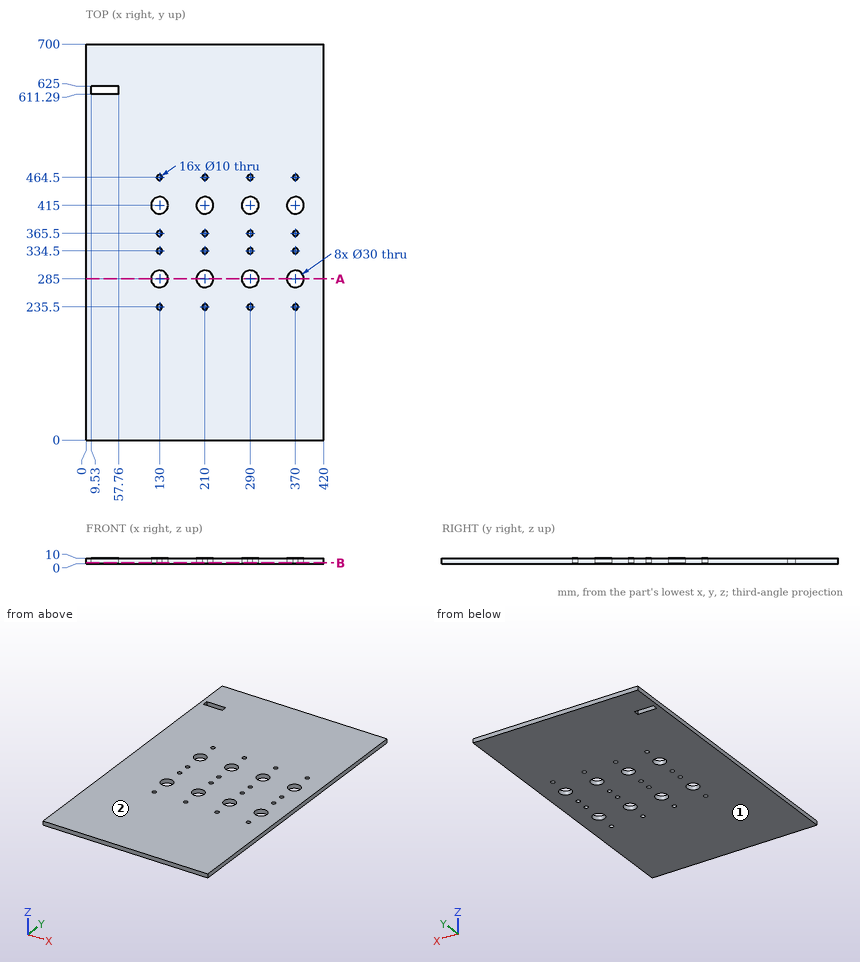
Answer from the drawing. Dimensions are ordinates in mm from the lowest x, y and z of the part. Give positions to 0.01 mm unless a question says otherwise; leave off trailing zeros. Order: outer loops, then holes, each group sorted by start corner. A loop starts at its lowest first (then second) coordinate and runs counter-clockwise, first axis right, second up.
Item 1: The part is cut by section A-A, the plane y = 285. Give the vertices of the cut face in (x, z), and give its area (3 significant figures).
From the geometry:
outline: (0, 0) - (115, 0) - (115, 10) - (0, 10) - close; (145, 0) - (195, 0) - (195, 10) - (145, 10) - close; (225, 0) - (275, 0) - (275, 10) - (225, 10) - close; (305, 0) - (355, 0) - (355, 10) - (305, 10) - close; (385, 0) - (420, 0) - (420, 10) - (385, 10) - close
area: 3,000 mm2
Item 2: For a pull along Z with two mould halves and no side action, classify the marked faces 1 and 2 as pulls with the +Z half, pulls with the -Z half, needs draft (parallel to the pull), parting line crosses it, or undercut.
From the geometry:
face 1: pulls with the -Z half
face 2: pulls with the +Z half
Item 3: Find the intervals of material crossed by probe 1 along X at (y, z) = (334.5, 2.5); probe 2 along Y at (x, z) = (277.5, 7); probe 3 along Y at (x, z) = (118, 4.5), in increasing order.
From the geometry:
probe 1: x = 0 to 125, 135 to 205, 215 to 285, 295 to 365, 375 to 420
probe 2: y = 0 to 276.71, 293.29 to 406.71, 423.29 to 700
probe 3: y = 0 to 276, 294 to 406, 424 to 700
Item 4: The part is cut by section B-B, the plane z = 2. Count the separate pieces of the cut face and the enclosed holes in it, and give its area (3 significant figures).
From the geometry:
separate pieces: 1
enclosed holes: 25
area: 286,000 mm2
